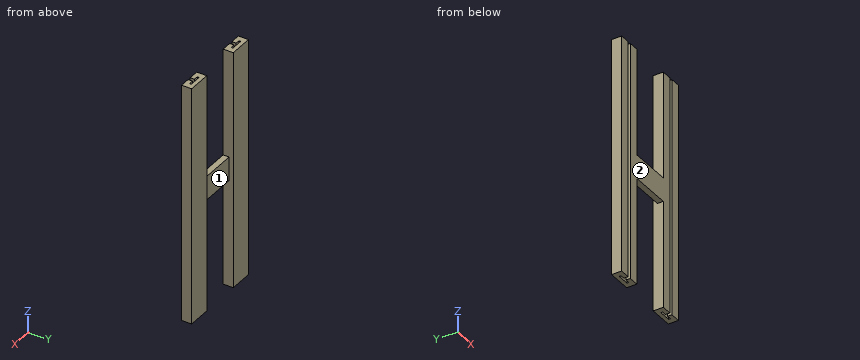
```python
from build123d import *

# Parameters (mm, degrees)
BOSS_EXTRUDE1_DEPTH     = 17
SKETCH2_W               = 70
SKETCH2_H               = 40
CUT_EXTRUDE1_DEPTH      = 7
CUT_EXTRUDE2_DEPTH      = 401.331856029
SKETCH4_W               = 150
SKETCH4_H               = 39.668143971
CUT_EXTRUDE3_DEPTH      = 1
CUT_EXTRUDE3_DEPTH_BACK = 18


with BuildPart() as part:
    # Sketch1 → Boss-Extrude1 (new body)
    with BuildSketch(Plane(origin=(0, 0, 0), x_dir=(1, 0, 0), z_dir=(0, 1, 0))):
        Polygon((40, 449.668143971), (40, 269.668143971), (110, 269.668143971), (110, 450), (150, 450), (150, 10), (110, 10), (110, 229.668143971), (40, 229.668143971), (40, 49.668143971), (0, 49.668143971), (0, 449.668143971), align=None)
    extrude(amount=BOSS_EXTRUDE1_DEPTH)

    # Sketch2 → Cut-Extrude1 (cut)
    with BuildSketch(Plane(origin=(0, 17, 0), x_dir=(1, 0, 0), z_dir=(0, 1, 0))):
        with Locations((75, 249.668143971)):
            Rectangle(SKETCH2_W, SKETCH2_H)
    extrude(amount=-CUT_EXTRUDE1_DEPTH, mode=Mode.SUBTRACT)

    # Sketch3 → Cut-Extrude2 (cut, through all)
    with BuildSketch(Plane.XY.offset(-49.668143971)):
        Polygon((17.25, 0), (17.25, 7.25), (9.75, 7.25), (9.75, 10.25), (30.25, 10.25), (30.25, 7.25), (22.75, 7.25), (22.75, 0), align=None)
    cut_extrude2 = extrude(amount=-CUT_EXTRUDE2_DEPTH, mode=Mode.SUBTRACT)

    # Mirror1: Cut-Extrude2 across plane
    add(cut_extrude2.mirror(Plane(origin=(75, 0, 0), x_dir=(0, 0, 1), z_dir=(1, 0, 0))), mode=Mode.SUBTRACT)

    # Sketch4 → Cut-Extrude3 (cut, two sides)
    with BuildSketch(Plane(origin=(0, 17, 0), x_dir=(1, 0, 0), z_dir=(0, 1, 0))) as cut_extrude3_sk:
        with Locations((75, 29.834071986)):
            Rectangle(SKETCH4_W, SKETCH4_H)
    extrude(amount=CUT_EXTRUDE3_DEPTH, mode=Mode.SUBTRACT)
    extrude(cut_extrude3_sk.sketch, amount=-CUT_EXTRUDE3_DEPTH_BACK, mode=Mode.SUBTRACT)


solid = part.part
```
Build history of the part. All positions in model axes, mm. Face numbers are marked on the shaded views. Give positions to 0.01 mm unless a question says otherwise; leave off trailing zeros. Order: outer loops, then holes, each group sorted by start corner. A loop starts at its lowest first (then second) coordinate and runs counter-clockwise, first axis right, second up. Notation, with made-up numbers: M 30,22.5 L 79,22.5 A22 cw 79,35.5 Z; hole C 71.25,-35 d7. An arc over 180 degrees is marked long. Return JSON: item names as keys, results as strings.
Q1. Wall check: probe 1 along X at (y, z) = (4, -412); probe 2 along X at (y, z) = (9, -282); probe 3 along X at (y, z) = (12.75, -149.5). Give the ranges that are in metal, low to high. Write a range as from..to.
Answer list:
{"probe 1": "x = 0..17.25, 22.75..40, 110..127.25, 132.75..150", "probe 2": "x = 0..9.75, 30.25..40, 110..119.75, 140.25..150", "probe 3": "x = 0..40, 110..150"}
Q2. Two-plate mould, pull along X, no slides. Class the marked faces 1 and 2: pulls with the +X half, pulls with the -X half, needs draft (parallel to the pull), parting line crosses it, or undercut.
Answer list:
{"face 1": "undercut", "face 2": "needs draft"}
Q3. Flat gauge pins, fed straight in: pin 1 (8 mm diameter, centred on x = 104, y = 6.5, fed in from -Z); pin 2 (8 mm diameter, centred on x = 68.5, y = 3, fed in from +Z); pin 3 (12 mm diameter, centred on x = 88.5, z = -241.5, fed in from +Y). Where does each tip first touch, or does it go through?
Answer list:
{"pin 1": "stops at z = -269.67", "pin 2": "stops at z = -229.67", "pin 3": "stops at y = 10"}
Q4. Band-saw the part on C-C (z = -249). Give the cut face in (x, y).
Answer list:
{"outline": "M 0,0 L 17.25,0 L 17.25,7.25 L 9.75,7.25 L 9.75,10.25 L 30.25,10.25 L 30.25,7.25 L 22.75,7.25 L 22.75,0 L 127.25,0 L 127.25,7.25 L 119.75,7.25 L 119.75,10.25 L 140.25,10.25 L 140.25,7.25 L 132.75,7.25 L 132.75,0 L 150,0 L 150,17 L 110,17 L 110,10 L 40,10 L 40,17 L 0,17 Z"}
Q5. Band-saw the part on D-D (x = 68). Give the cut face in (y, z), then the cut area to 3 significant figures.
Answer list:
{"outline": "M 0,-269.67 L 10,-269.67 L 10,-229.67 L 0,-229.67 Z", "area": "400 mm^2"}
Q6. Band-saw the part on A-A (z = -120). Give the cut face in (x, y).
Answer list:
{"outline": "M 0,0 L 17.25,0 L 17.25,7.25 L 9.75,7.25 L 9.75,10.25 L 30.25,10.25 L 30.25,7.25 L 22.75,7.25 L 22.75,0 L 40,0 L 40,17 L 0,17 Z; M 110,0 L 127.25,0 L 127.25,7.25 L 119.75,7.25 L 119.75,10.25 L 140.25,10.25 L 140.25,7.25 L 132.75,7.25 L 132.75,0 L 150,0 L 150,17 L 110,17 Z"}
Q7. Band-saw the part on B-B (y = 13.25). Give the cut face in (x, z).
Answer list:
{"outline": "M 0,-449.67 L 40,-449.67 L 40,-49.67 L 0,-49.67 Z; M 110,-450 L 150,-450 L 150,-49.67 L 110,-49.67 Z"}
